```python
from build123d import *
from build123d.topology import SkipClean

# Parameters (mm, degrees)
SKETCH1_W                  = 20
SKETCH1_H                  = 30
BOSS_EXTRUDE1_DEPTH        = 3
F_3_2_3_2_DIAMETER_HOLE1_D = 3.2
SKETCH5_R                  = 3
SKETCH5_R_2                = 1.6
BOSS_EXTRUDE2_DEPTH        = 20
SKETCH6_R                  = 2.75
CUT_EXTRUDE1_DEPTH         = 27.925824036
SKETCH7_W                  = 20
SKETCH7_H                  = 40
CUT_EXTRUDE2_DEPTH         = 34.970575503
FILLET1_R                  = 3


with BuildPart() as part:
    # Sketch1 → Boss-Extrude1 (new body)
    with BuildSketch(Plane.XY):
        Rectangle(SKETCH1_W, SKETCH1_H)
    extrude(amount=BOSS_EXTRUDE1_DEPTH)

    # 3.2 _3.2_ Diameter Hole1 (through all)
    with Locations(Plane.XY.offset(3)):
        with Locations((-6.5, 11.5), (6.5, 11.5), (6.5, -11.5), (-6.5, -11.5)):
            Hole(F_3_2_3_2_DIAMETER_HOLE1_D / 2)

    # Sketch5 → Boss-Extrude2 (add)
    # profile 1 of 4: a face of its own
    with SkipClean():  # the faces are left unmerged after this step: merging them gives an invalid solid
        with BuildSketch(Plane.XY.offset(3)):
            with Locations(Location((-6.5, 11.5, 0), (0, 0, 180))):
                Circle(SKETCH5_R)
            with Locations((-6.5, 11.5)):
                Circle(SKETCH5_R_2, mode=Mode.SUBTRACT)
        # profile 2 of 4: a face of its own
        with BuildSketch(Plane.XY.offset(3)):
            with Locations(Location((6.5, 11.5, 0), (0, 0, 180))):
                Circle(SKETCH5_R)
            with Locations((6.5, 11.5)):
                Circle(SKETCH5_R_2, mode=Mode.SUBTRACT)
        # profile 3 of 4: a face of its own
        with BuildSketch(Plane.XY.offset(3)):
            with Locations(Location((6.5, -11.5, 0), (0, 0, 180))):
                Circle(SKETCH5_R)
            with Locations((6.5, -11.5)):
                Circle(SKETCH5_R_2, mode=Mode.SUBTRACT)
        # profile 4 of 4: a face of its own
        with BuildSketch(Plane.XY.offset(3)):
            with Locations(Location((-6.5, -11.5, 0), (0, 0, 180))):
                Circle(SKETCH5_R)
            with Locations((-6.5, -11.5)):
                Circle(SKETCH5_R_2, mode=Mode.SUBTRACT)
        extrude(amount=BOSS_EXTRUDE2_DEPTH)
    add(part.part.scale(1), mode=Mode.REPLACE)  # the faces are merged on a copy

    # Sketch6 → Cut-Extrude1 (cut, through all)
    with BuildSketch(Plane.XY.offset(3)):
        Circle(SKETCH6_R)
    extrude(amount=-CUT_EXTRUDE1_DEPTH, mode=Mode.SUBTRACT)

    # Sketch7 → Cut-Extrude2 (cut, through all)
    with BuildSketch(Plane(origin=(10, 0, 0), x_dir=(0, 0, -1), z_dir=(1, 0, 0))):
        with Locations((-20, 0)):
            Rectangle(SKETCH7_W, SKETCH7_H)
    extrude(amount=-CUT_EXTRUDE2_DEPTH, mode=Mode.SUBTRACT)

    # Fillet1
    fillet1_edges = [part.edges().sort_by_distance(p)[0] for p in [
        (10, -15, 1.5),
        (-10, -15, 1.5),
        (-10, 15, 1.5),
        (10, 15, 1.5),
    ]]
    fillet(fillet1_edges, radius=FILLET1_R)


solid = part.part
```
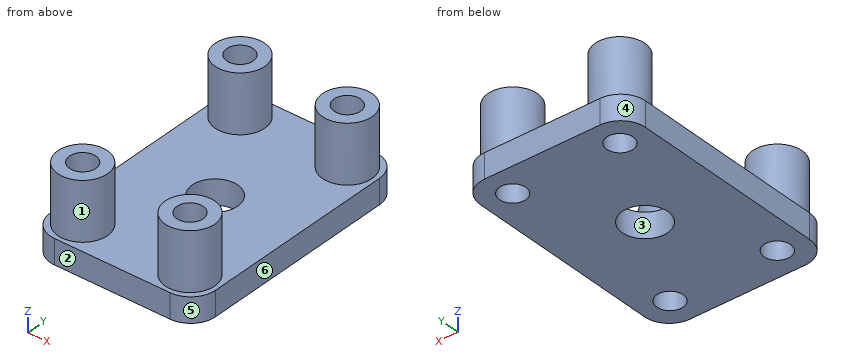
Read the model definition and answer for the solid it produces. Units are mm, in the model's axes. Face numbers are marked on the shaded views. A direction names the side the tool comes from. Coordinates: 2 decimals unless noted, no trailing zeros. Loops run counter-clockwise (first coordinate to the right, second up) from the corner with the lowest first, then second, coordinate; pieces in that order, holes last. Notation, with made-up numbers: (9.5, 63) -> (21.5, 63) arc R12 ccw to (21.5, 82) -> close; hole circle Ø9 at (-24.5, 28). An arc over 180 degrees is marked (long way). Return JSON: item names as keys, results as strings.
Item 1: For a pull along Y with two mould halves and no side action, classify the marked faces 3, 4, 5 and 6 as +Y half, -Y half, draft (parallel to the pull), parting line (faces both ways), or undercut.
Answers:
{"face 3": "undercut", "face 4": "+Y half", "face 5": "-Y half", "face 6": "draft"}
Item 2: Find section D-D (y = 0). Determine the outline of the cut face in (x, z), plus the area to 3 significant figures.
Answers:
{"outline": "(-10, 0) -> (-2.75, 0) -> (-2.75, 3) -> (-10, 3) -> close; (2.75, 0) -> (10, 0) -> (10, 3) -> (2.75, 3) -> close", "area": "43.5 mm2"}
Item 3: Find the intervals of material crossed by probe 1 along Y at (x, z) = (6.5, 5.75); probe 2 along X at (y, z) = (11.5, 2.15); probe 3 along Y at (x, z) = (0, 1.7), in increasing order.
Answers:
{"probe 1": "y = -14.5 to -13.1, -9.9 to -8.5, 8.5 to 9.9, 13.1 to 14.5", "probe 2": "x = -10 to -8.1, -4.9 to 4.9, 8.1 to 10", "probe 3": "y = -15 to -2.75, 2.75 to 15"}
Item 4: For the marked faces 1 and 2, determine the directions among +Z, -Z, +X, -X, +Y, -Y from which every point of the face is accessible in a straight line to the end or side of a thin tool.
Answers:
{"face 1": "+Z", "face 2": "+Z, -Z, +X, -X, -Y"}
Item 5: Flat-ended cylindrical pins translate along their axes: P1, Ø1.9, axis at x = -6.5, y = 11.5, coming from the +Z side; P2, Ø8, axis at x = 3.5, y = 7.5, coming from the +Z side; P3, Ø7, axis at x = 0, y = 0, coming from the +Z side; P4, Ø1.5, axis at x = -5.5, z = 5, coming from the -Y side. Find the tip coordinate at first contact, or state that the pin passes through.
Answers:
{"P1": "passes through", "P2": "stops at z = 10", "P3": "stops at z = 3", "P4": "stops at y = -14.49"}
Item 6: Find section C-C (x = 0). Determine the outline of the cut face in (y, z).
Answers:
{"outline": "(-15, 0) -> (-2.75, 0) -> (-2.75, 3) -> (-15, 3) -> close; (2.75, 0) -> (15, 0) -> (15, 3) -> (2.75, 3) -> close"}
Item 7: Find section B-B (y = -11.5). Determine the outline of the cut face in (x, z).
Answers:
{"outline": "(-10, 0) -> (-8.1, 0) -> (-8.1, 10) -> (-9.5, 10) -> (-9.5, 3) -> (-10, 3) -> close; (-4.9, 0) -> (4.9, 0) -> (4.9, 10) -> (3.5, 10) -> (3.5, 3) -> (-3.5, 3) -> (-3.5, 10) -> (-4.9, 10) -> close; (8.1, 0) -> (10, 0) -> (10, 3) -> (9.5, 3) -> (9.5, 10) -> (8.1, 10) -> close"}
Item 8: Find section A-A (z = 3.75). Determine the outline of the cut face in (x, y), plus the area to 3 significant figures.
Answers:
{"outline": "circle Ø6 at (-6.5, -11.5); circle Ø6 at (-6.5, 11.5); circle Ø6 at (6.5, -11.5); circle Ø6 at (6.5, 11.5); hole circle Ø3.2 at (-6.5, -11.5); hole circle Ø3.2 at (-6.5, 11.5); hole circle Ø3.2 at (6.5, -11.5); hole circle Ø3.2 at (6.5, 11.5)", "area": "80.9 mm2"}
